Build history of the part. All positions in model axes, mm. A direction names the side the tool comes from. Round coordinates to 2 decimals unless told otherwise and drop trailing zeros. Write each loop counter-clockwise with the first axis right and the second up, starting at its lowest first coordinate (ties: lowest second). Pieces come first, ordered by that corner, then holes. Notation, with made-up numbers: (-25.75, 83.25) - (-7.75, 83.25) arc R25 ccw to (-7.75, 100.25) - close; hole circle Ø11 at (31.5, -4.75). An arc over 180 degrees is marked (long way). Write each question's results on one line, items separated by ' | '.
Autodesk Inventor part; units mm, degrees
ref_plane "Work Plane1" through (33.5, 0, 0) normal (1, 0, 0) x (0, 1, 0)
ref_plane "XZ Plane" through (0, 0, 0) normal (0, 1, 0) x (-1, 0, 0)
ref_plane "XY Plane" through (0, 0, 0) normal (0, 0, 1) x (1, 0, 0)
sketch "Sketch1" plane through (0, 0, 0) normal (0, 1, 0) x (-1, 0, 0)
  circle A0 centre (0, 0) radius 33.5
  dimension "d0" = 67
extrude "Extrusion1" add sketch "Sketch1" along normal blind 5
ref_plane "Work Plane1" through (33.5, 0, 0) normal (1, 0, 0) x (0, 1, 0)
sketch "Sketch2" plane through (33.5, 0, 0) normal (1, 0, 0) x (0, 1, 0)
  line L0 (0, -33.5) -> (0, 33.5)
  point P0 (0, 0)
  point P1 (2.5, 0)
  dimension "d4" = 2.5
hole "Hole1" at (33.5, 2.5, 0) direction (-1, 0, 0) diameter 2.5 depth 8 tip angle 118
pattern_circular "Circular Pattern1" count 3 over 360 about axis through (0, 0, 0) along (0, 1, 0) of "Hole1"
sketch "Sketch3" plane through (0, 0, 0) normal (0, -1, 0) x (1, 0, 0)
  point P0 (0, 0)
  point P1 (0, 0)
hole "Hole2" at (0, 0, 0) direction (0, 1, 0) diameter 5 depth 8 tip angle 118
properties part number "Engine bulkhead" material "Steel AISI 1006 85 HR"
(1) Drill centre line: probe 1 along X at (y, z) = (3.8, 0). Where is it in solid material? Low to high. Write a range as [from, to].
Worked answers:
probe 1: x = [-33.5, -2.5], [2.5, 33.5]
(2) Slice it at A-A, the plane x = 0. Write the cut outline in (y, z).
Worked answers:
outline: (0, -33.5) - (5, -33.5) - (5, -2.5) - (0, -2.5) - close; (0, 2.5) - (5, 2.5) - (5, 33.5) - (0, 33.5) - close
(3) Tool access for faces 1 (the cylindrical face through (7.262, 2.465, 32.703)), 2 (the conical face through (-12.464, 2.715, 21.532)), 3 (the cylindrical face through (29.44, 1.26, 0.16)): list every direction of +Z, -Z, +X, -X, +Y, -Y with a clear straight run to the whole face (end or side of a thin tool).
Worked answers:
face 1: +Y, -Y | face 2: none | face 3: +X
(4) Two-plate mould, pull along Y, no slides. Class faces 4 (the flat face through (0, 5, -7)), 5 (the cylindrical face through (-13.64, 2.45, -26.12)), 6 (the cylindrical face through (2.44, 2.54, 0.54)): released by +Y, released by -Y, zero draft, split by the parting line, or undercut.
Worked answers:
face 4: released by +Y | face 5: undercut | face 6: zero draft
(5) Slice it at C-C, the plane z = -15.5. Write the cut outline in (x, y).
Worked answers:
outline: (-29.7, 0) - (29.7, 0) - (29.7, 5) - (-29.7, 5) - close
(6) Flat gauge pins, fed straight in: pin 1 Ø1.5 at (y, z) = (2.5, 0) entering from +X; pin 2 Ø3 at (y, z) = (1.5, 16) entering from +X; pin 3 Ø3 at (x, z) = (0, 0) entering from +Y; pin 4 Ø1 at (y, z) = (1.5, -6) entering from -X. Where does each tip first touch, or does it go through?
Worked answers:
pin 1: stops at x = 25.2 | pin 2: stops at x = 30.2 | pin 3: passes through | pin 4: stops at x = -33.05
(7) Slice it at D-D, the plane x = -26. Write the cut outline in (y, z).
Worked answers:
outline: (0, -21.12) - (5, -21.12) - (5, 21.12) - (0, 21.12) - close
(8) Slice it at B-B, the plane x = 29.5. Write the cut outline in (y, z).
Worked answers:
outline: (0, -15.87) - (5, -15.87) - (5, 15.87) - (0, 15.87) - close; hole circle Ø2.5 at (2.5, 0)
